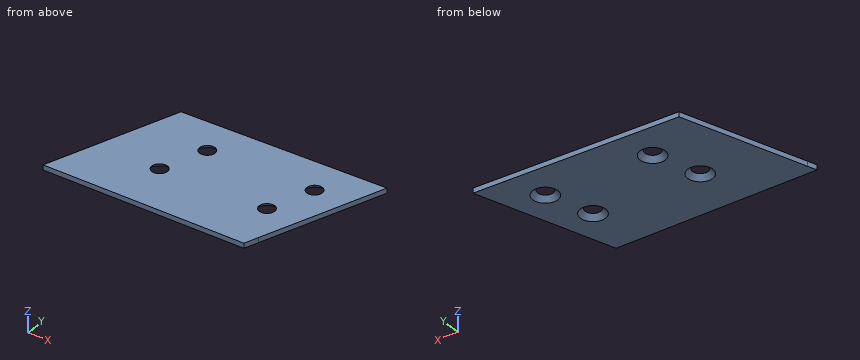
from build123d import *

# Parameters (mm, degrees)
BOSS_EXTRUDE1_DEPTH                            = 2
BOSS_EXTRUDE2_DEPTH                            = 2
SKETCH4_R                                      = 2.5
CUT_EXTRUDE2_DEPTH                             = 2
CSK_FOR_M5_FLAT_HEAD_MACHINE_SCREW1_AT_2_COUNT = 2
CSK_FOR_M5_FLAT_HEAD_MACHINE_SCREW1_AT_2_PITCH = 44.45
CSK_FOR_M5_FLAT_HEAD_MACHINE_SCREW1_AT_3_COUNT = 2
CSK_FOR_M5_FLAT_HEAD_MACHINE_SCREW1_AT_3_PITCH = 54.156278026
CSK_FOR_M5_FLAT_HEAD_MACHINE_SCREW1_AT_4_COUNT = 2
CSK_FOR_M5_FLAT_HEAD_MACHINE_SCREW1_AT_4_PITCH = 20


with BuildPart() as part:
    # Sketch2 → Boss-Extrude1 (new body)
    with BuildSketch(Plane.XY):
        Polygon((-54.61917065, -24.589230235), (30.72482935, -24.589230235), (13.852659447, -75.725684813), (-71.491340553, -75.725684813), align=None)
    extrude(amount=BOSS_EXTRUDE1_DEPTH)

    # Sketch3 → Boss-Extrude2 (add)
    with BuildSketch(Plane.XY.offset(2)):
        Polygon((-72.764711867, -79.585039875), (11.90144755, -81.639450446), (13.852659447, -75.725684813), (-71.491340553, -75.725684813), align=None)
    extrude(amount=-BOSS_EXTRUDE2_DEPTH)

    # Sketch4 → Cut-Extrude2 (cut)
    with BuildSketch(Plane.XY.offset(2)):
        with Locations((-32.900665919, -39.829230235)):
            Circle(SKETCH4_R)
        with Locations((11.549334081, -39.829230235)):
            Circle(SKETCH4_R)
        with Locations((5.282742972, -58.822119322)):
            Circle(SKETCH4_R)
        with Locations((-39.167257028, -58.822119322)):
            Circle(SKETCH4_R)
    extrude(amount=-CUT_EXTRUDE2_DEPTH, mode=Mode.SUBTRACT)

    # Sketch5 → CSK for M5 Flat Head Machine Screw1 (revolve, cut)
    with BuildSketch(Plane(origin=(11.549334081, -39.829230235, 0), x_dir=(0, 1, 0), z_dir=(1, 0, 0))):
        Polygon((0, 0), (0, 2), (2.75, 2), (2.75, 2.45), (5.2, 0), align=None)
    csk_for_m5_flat_head_machine_screw1 = revolve(axis=Axis((11.549334081, -39.829230235, -6.35), (0, 0, 1)), mode=Mode.SUBTRACT)

    # CSK for M5 Flat Head Machine Screw1 at 2: CSK for M5 Flat Head Machine Screw1 ×2
    with Locations(*[(-i * CSK_FOR_M5_FLAT_HEAD_MACHINE_SCREW1_AT_2_PITCH, 0, 0) for i in range(1, CSK_FOR_M5_FLAT_HEAD_MACHINE_SCREW1_AT_2_COUNT)]):
        add(csk_for_m5_flat_head_machine_screw1, mode=Mode.SUBTRACT)

    # CSK for M5 Flat Head Machine Screw1 at 3: CSK for M5 Flat Head Machine Screw1 ×2
    with Locations(*[Vector(-0.9364859063085671, -0.35070521422616713, 0) * (i * CSK_FOR_M5_FLAT_HEAD_MACHINE_SCREW1_AT_3_PITCH) for i in range(1, CSK_FOR_M5_FLAT_HEAD_MACHINE_SCREW1_AT_3_COUNT)]):
        add(csk_for_m5_flat_head_machine_screw1, mode=Mode.SUBTRACT)

    # CSK for M5 Flat Head Machine Screw1 at 4: CSK for M5 Flat Head Machine Screw1 ×2
    with Locations(*[Vector(-0.31332955547970937, -0.9496444543421964, 0) * (i * CSK_FOR_M5_FLAT_HEAD_MACHINE_SCREW1_AT_4_PITCH) for i in range(1, CSK_FOR_M5_FLAT_HEAD_MACHINE_SCREW1_AT_4_COUNT)]):
        add(csk_for_m5_flat_head_machine_screw1, mode=Mode.SUBTRACT)


solid = part.part
Verification items for the finished model (mm, model axes). Round coordinates to 2 decimals unless told otherwise and drop trailing zeros. Loops run counter-clockwise (first coordinate to the right, second up) from the corner with the lowest first, then second, coordinate; pieces in that order, holes last. Notation, with made-up numbers: (-29.75, 19.5) - (14.25, 19.5) arc R16 cw to (14.25, 31.5) - close; hole circle Ø1 at (1, 47). An arc over 180 degrees is marked (long way). Answer in a Markdown table with one row per item. Add a question column.
Q1. Section check D-D on y = -60. State how many separate pieces and enclosed holes the cut face has, plus the area to 3 significant figures.
Q2. Gauge pin test, flat end, axial feed: pin 1 (1 mm diameter, centred on x = -21, z = 0.5, fed in from -Y). Record the tip position at first contact, or that the pin passes through.
Q3. Section check A-A on z = 1.6. Enter the section's corners in (x, y), plus the area to 3 significant figures.
Q4. Section check B-B on y = -74.5. Enter the section's corners in (x, z).
Q5. Section check C-C on x = 19. Enter the section's corners in (y, z).
Q6. Material ranges on line 1 (X direction, y = -41, z = 0.9); line 2 (Y direction, x = 9, z = 0.85); line 3 (X direction, y = -43.5, z = 0.85), recorded low to high.
Found:
| question | item | result |
|---|---|---|
| 1 | separate pieces | 3 |
| 1 | enclosed holes | 0 |
| 1 | area | 138 mm² |
| 2 | pin 1 | stops at y = -80.85 |
| 3 | outline | (-72.76, -79.59) - (11.9, -81.64) - (30.72, -24.59) - (-54.62, -24.59) - close; hole circle Ø7.2 at (-39.17, -58.82); hole circle Ø7.2 at (-32.9, -39.83); hole circle Ø7.2 at (5.28, -58.82); hole circle Ø7.2 at (11.55, -39.83) |
| 3 | area | 4,620 mm² |
| 4 | outline | (-71.09, 0) - (14.26, 0) - (14.26, 2) - (-71.09, 2) - close |
| 5 | outline | (-60.13, 0) - (-24.59, 0) - (-24.59, 2) - (-60.13, 2) - close |
| 6 | line 1 | x = -60.03 to -37.04, -28.76 to 7.41, 15.69 to 25.31 |
| 6 | line 2 | y = -81.57 to -61.08, -56.56 to -43.35, -36.3 to -24.59 |
| 6 | line 3 | x = -60.86 to -35.23, -30.57 to 9.22, 13.88 to 24.49 |
